For this review, use the dimensioned drawing (mm, ordinates from the lowest corner) and the shaded views. Give positions to 0.01 mm unless a question says otherwise; leave off trailing zeros. Loops run counter-clockwise (first coordinate to the right, second up) from the corner with the lowest first, then second, coordinate; pieces in that order, holes last. Notation, with made-up numbers: M 16,24 L 34,24 A30 ccw 34,46 Z; hole C 50,-31 d2. An arc over 180 degrees is marked long. Use one line per item in the form item = value. Start each with the question number.
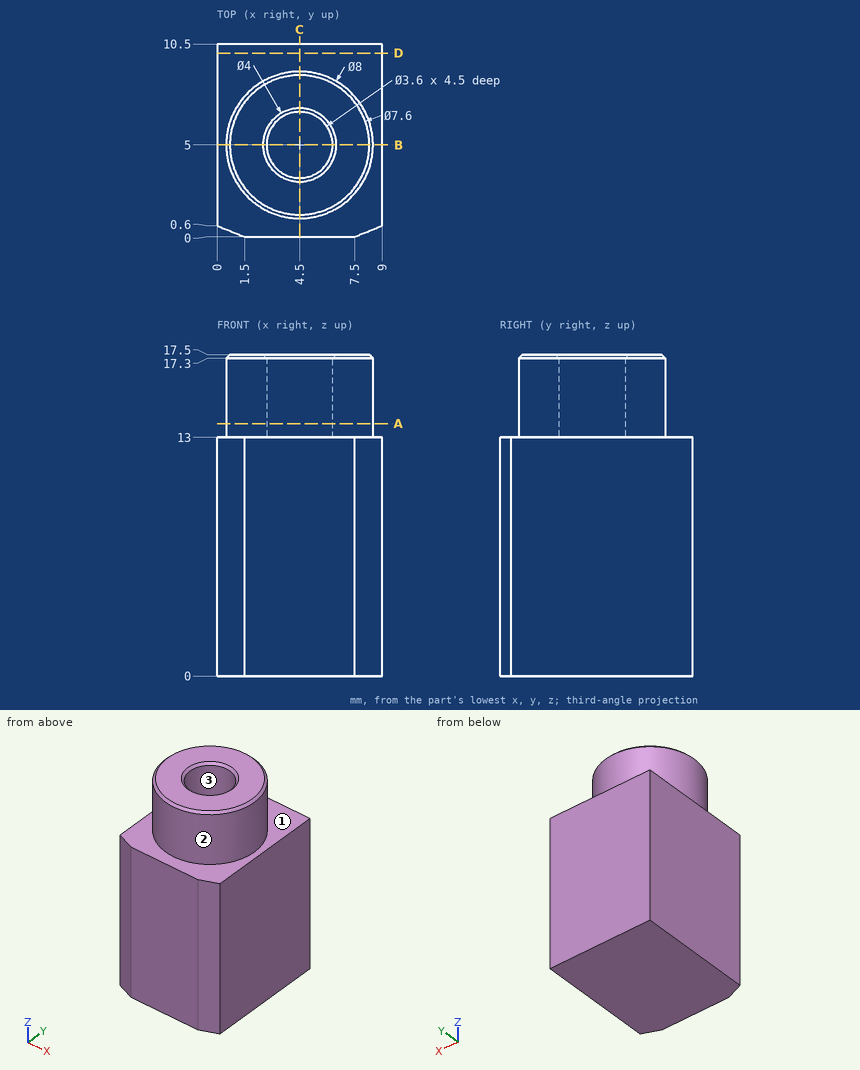
Q1. Clearance check with flat-ended pins moving along their axes: pin 1 Ø5 at (x, y) = (2.5, 1.5) entering from -Z; pin 2 Ø3 at (x, y) = (4.5, 5) entering from +Z. State where each tip first meets the part, or that it passes through.
Q2. Take a section at A-A on z = 13.75. Give the boundary of the cut face in (x, y).
Q3. Take a section at D-D on y = 10. Give the boundary of the cut face in (x, z), plus the area to 3 significant figures.
Q4. The part is to be moulded in two halves that separate along Y. For the marked faces 1, 2 and 3, say which applies: pulls with the +Y half, pulls with the -Y half, needs draft (parallel to the pull), parting line crosses it, or undercut.
Q5. Take a section at C-C on x = 4.5. Give the boundary of the cut face in (y, z), plus the area to 3 significant figures.
Q6. Wall thickness on probe 1 along Y at (x, z) = (4.5, 15.3); probe 2 along Z at (x, y) = (8.5, 7); probe 3 along X at (y, z) = (6.5, 15.5): over which ranges is each line inside the solid? List them lowest first.
Q7. Take a section at B-B on y = 5. Give the boundary of the cut face in (x, z), plus the area to 3 significant figures.
Response values:
q1.pin_1 = 0
q1.pin_2 = 13
q2.outline = C 4.5,5 d8; hole C 4.5,5 d3.6
q3.outline = M 0,0 L 9,0 L 9,13 L 0,13 Z
q3.area = 117 mm^2
q4.face_1 = needs draft
q4.face_2 = parting line crosses it
q4.face_3 = undercut
q5.outline = M 0,0 L 10.5,0 L 10.5,13 L 9,13 L 9,17.3 L 8.8,17.5 L 7,17.5 L 6.8,17.3 L 6.8,13 L 3.2,13 L 3.2,17.3 L 3,17.5 L 1.2,17.5 L 1,17.3 L 1,13 L 0,13 Z
q5.area = 156 mm^2
q6.probe_1 = 1 to 3.2, 6.8 to 9
q6.probe_2 = 0 to 13
q6.probe_3 = 0.79 to 3.51, 5.49 to 8.21
q7.outline = M 0,0 L 9,0 L 9,13 L 8.5,13 L 8.5,17.3 L 8.3,17.5 L 6.5,17.5 L 6.3,17.3 L 6.3,13 L 2.7,13 L 2.7,17.3 L 2.5,17.5 L 0.7,17.5 L 0.5,17.3 L 0.5,13 L 0,13 Z
q7.area = 137 mm^2
